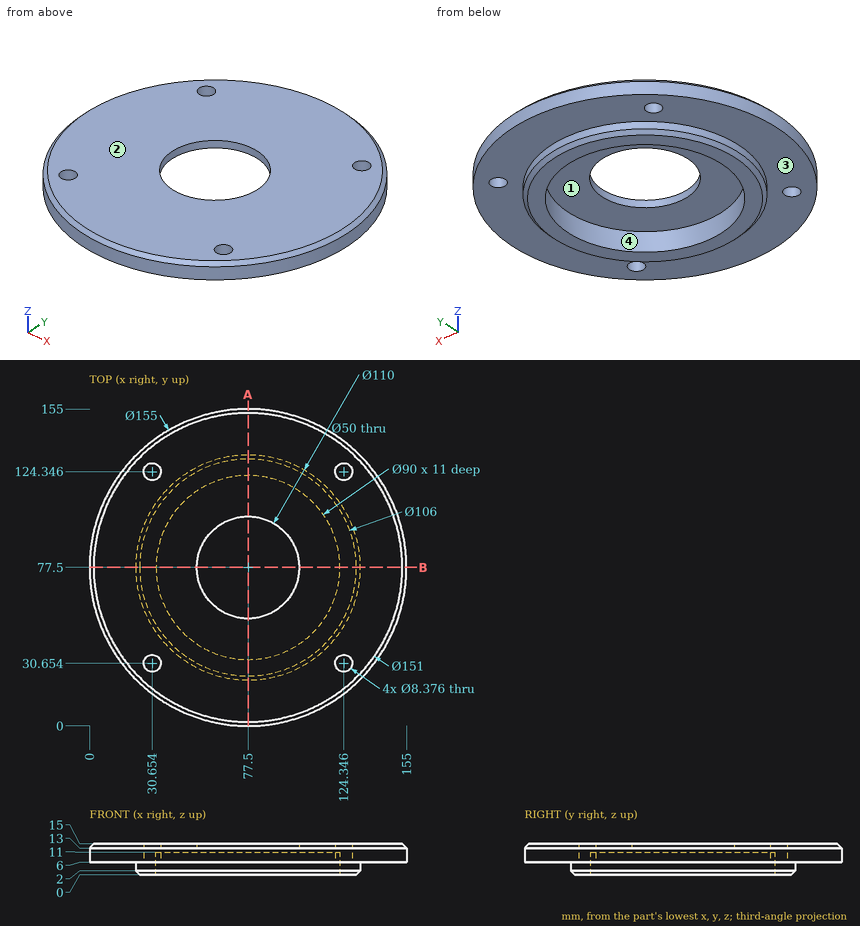
Geometry check sheet. Reference: drawing and pictorial views, mm from the part's lowest x, y, z. A direction names the side the tool comes from. Round coordinates to 2 decimals unless told otherwise and drop trailing zeros. Loops run counter-clockwise (first coordinate to the right, second up) from the corner with the lowest first, then second, coordinate; pieces in that order, holes last. Notation, with made-up numbers: (-36, 55.5) - (2, 55.5) arc R21 ccw to (2, 94.5) - close; hole circle Ø11 at (35.25, 7). An arc over 180 degrees is marked (long way). Write item = value, one per line. Start each with the question number.
Q1. Release check for a two-part mould opening along Y. For the marked faces 3 and 4 record: pulls with the +Y half, pulls with the -Y half, needs draft (parallel to the pull), parting line crosses it, or undercut.
Q2. Access from +Z, -Z, +X, -X, +Y, -Y to the whole of each face (thin tool, end or side, straight path). Record for the marked faces 1 and 2.
Q3. Depth check by flat-ended pin: P1, Ø6, axis at x = 96, z = 9, coming from the +Y side; P2, Ø13.5, axis at x = 124.35, y = 30.65, coming from the +Z side; P3, Ø13.5, axis at x = 30.65, y = 30.65, coming from the -Z side; P4, Ø6, axis at y = 116.5, z = 12.5, coming from the -X side. Enter the tip coordinate at first touch or a pass-through.
Q4. Thickness scan on L1, parallel to Y at x = 77.5, z = 8; L2, parallel to Y at x = 123, z = 13.5; L3, parallel to Z at x = 21, y = 117.5. Record the ranges inside material, lowest first.
Q5. Section check A-A (x = 77.5). Record the boundary of the cut face in (y, z).
Derived:
q1.face_3 = needs draft
q1.face_4 = undercut
q2.face_1 = -Z
q2.face_2 = +Z, +X, -X, +Y, -Y
q3.P1 = 153.43
q3.P2 = 15
q3.P3 = 6
q3.P4 = 8.87
q4.L1 = 0 to 32.5, 122.5 to 155
q4.L2 = 15.38 to 26.69, 34.62 to 120.38, 128.31 to 139.62
q4.L3 = 6 to 15
q5.outline = (0, 6) - (22.5, 6) - (22.5, 2) - (24.5, 0) - (32.5, 0) - (32.5, 11) - (52.5, 11) - (52.5, 15) - (2, 15) - (0, 13) - close; (102.5, 11) - (122.5, 11) - (122.5, 0) - (130.5, 0) - (132.5, 2) - (132.5, 6) - (155, 6) - (155, 13) - (153, 15) - (102.5, 15) - close
